Can you work these out from the model? Positions are in its coordinate system, mm. A direction names the side the tool comes from. Coordinates: 2 decimals unless noted, no trailing zeros. Write each loop counter-clockwise with the first axis right and the second up, starting at its lowest first coordinate (ties: lowest second). Pieces come first, ordered by that corner, then holes. Notation, with made-up numbers: (-22.75, -27) - (17.25, -27) arc R10 cw to (17.25, -12) - close; hole circle Ø1 at (40, -1.75). An arc over 180 degrees is marked (long way). Use one line per item in the form item = value. Start each with the question number.
(1) If we section it at D-D on y = -57.5: Please give me the cut outline in (x, z), then the cut area to 3 significant figures.
(2) If we section it at B-B on x = 67.5: Please give me the cut outline in (y, z).
(3) On a 3-axis mill with a long thin cutter (end or side, diameter ignored), from which of +Z, -Z, +X, -X, +Y, -Y can I reach the whole of each face in a straight line? I mean faces 5 (the face through (102.8, -44.07, 0.02)), 6 (the face through (88.89, -38.34, 0.02)), 7 (the face through (76.481, -76.275, 0.022)). Say none if no direction works.
(4) Thinking about a two-plate mould opening in Y: for faces 1 (the face through (22.77, -84.54, 0.02)), 2 (the face through (126.226, -25.71, 0.022)), 3 (the face through (121.068, -37.137, 0.022)), 4 (the face through (108, 19, 1.588)), which applies, pulls with the +Y half, pulls with the -Y half, needs draft (parallel to the pull), parting line crosses it, or undercut?
(5) If we section it at A-A on z = -0.25: Please give me the cut outline in (x, y), then the cut area to 3 significant figures.
(6) If I drill on probe 1 along Y at (x, z) = (52, 0); probe 2 along Y at (x, z) = (72.5, 0.25); probe 3 along X at (y, z) = (-55, 0.55), over which ranges is the centre line in solid material (lowest first)? Write a range as from..to.
(7) For pin 1 Ø1.5 at (x, z) = (19.5, 1) entering from +Y; pin 2 Ø1 at (y, z) = (135, 0) entering from -X; pin 3 Ø1 at (x, z) = (1, 0.5) entering from +Y; pin 4 Ø8 at (x, y) = (44.5, 114) entering from +Z, each with a flat end and sliding along its axis, tell me the tip position at first contact or that it passes through.
(8) If we section it at C-C on x = 84.5: Please give me the cut outline in (y, z).
```python
from build123d import *

# Parameters (mm, degrees)
BOSS_EXTRUDE1_DEPTH = 1.5875
SKETCH3_W           = 208.645691316
SKETCH3_H           = 383.026987577
CUT_EXTRUDE1_DEPTH  = 121.098895727
BOSS_EXTRUDE2_DEPTH = 1.5875
FILLET1_R           = 6.35
FILLET2_R           = 12.7
SKETCH6_W           = 3.302
SKETCH6_H           = 12.7
CUT_EXTRUDE2_DEPTH  = 4.175


with BuildPart() as part:
    # Sketch2 → Boss-Extrude1 (new body, symmetric)
    with BuildSketch(Plane.XY):
        with BuildLine():
            ThreePointArc((-120.098895727, 19.05), (0.406748907, 139.2017743), (120.203613722, 18.343301545))
            ThreePointArc((120.203613722, 18.343301545), (101.067699546, -47.629728931), (50.138751442, -93.726))
            ThreePointArc((50.138751442, -93.726), (0.040174098, -101.514794876), (-50.058403246, -93.726))
            ThreePointArc((-50.058403246, -93.726), (-101.163912713, -47.327889321), (-120.098895727, 19.05))
        make_face()
        with BuildLine():
            ThreePointArc((-104.858895727, 19.05), (0.361930242, 123.961840203), (104.963877332, 18.432938489))
            ThreePointArc((104.963877332, 18.432938489), (88.446745877, -39.065849025), (44.40486057, -79.553359885))
            ThreePointArc((44.40486057, -79.553359885), (0.040463589, -86.274794876), (-44.323959374, -79.553531384))
            ThreePointArc((-44.323959374, -79.553531384), (-88.517658334, -38.801393502), (-104.858895727, 19.05))
        make_face(mode=Mode.SUBTRACT)
    extrude(amount=BOSS_EXTRUDE1_DEPTH, both=True)

    # Sketch3 → Cut-Extrude1 (cut, through all)
    with BuildSketch(Plane(origin=(0, 0, 0), x_dir=(0, 0, -1), z_dir=(1, 0, 0))):
        with Locations((4.266053154, 20.866300598)):
            Rectangle(SKETCH3_W, SKETCH3_H)
    extrude(amount=-CUT_EXTRUDE1_DEPTH, mode=Mode.SUBTRACT)

    # Sketch5 → Boss-Extrude2 (add, symmetric)
    with BuildSketch(Plane.XY):
        Polygon((106.258152496, -51.988683319), (130.011728615, -28.168431361), (114.573822099, -18.142937646), (100.046993583, -49.235229101), align=None)
    extrude(amount=BOSS_EXTRUDE2_DEPTH, both=True)

    # Fillet1
    fillet1_edges = [part.edges().sort_by_distance(p)[0] for p in [
        (100.046993583, -49.235229101, 0),
    ]]
    fillet(fillet1_edges, radius=FILLET1_R)

    # Fillet2
    fillet2_edges = [part.edges().sort_by_distance(p)[0] for p in [
        (114.573822099, -18.142937646, 0),
    ]]
    fillet(fillet2_edges, radius=FILLET2_R)

    # Sketch6 → Cut-Extrude2 (cut, through all)
    with BuildSketch(Plane.XY.offset(1.5875)):
        with Locations((1.651, 136.662280289)):
            Rectangle(SKETCH6_W, SKETCH6_H)
        Polygon((108.166218002, 79.740204673), (106.494925174, 82.588008087), (95.541835122, 76.159958748), (97.21312795, 73.312155334), align=None)
        Polygon((95.424252626, -39.741107061), (97.095545407, -36.89330362), (118.130209204, -49.237934313), (116.458916422, -52.085737754), align=None)
        with Locations((1.651, -98.974789488)):
            Rectangle(SKETCH6_W, SKETCH6_H)
    extrude(amount=-CUT_EXTRUDE2_DEPTH, mode=Mode.SUBTRACT)


solid = part.part
```
Reported:
q1.outline = (74.16, -1.59) - (94.22, -1.59) - (94.22, 1.59) - (74.16, 1.59) - close
q1.area = 63.7 mm2
q2.outline = (-83.33, -1.59) - (-63.89, -1.59) - (-63.89, 1.59) - (-83.33, 1.59) - close; (99.41, -1.59) - (118.49, -1.59) - (118.49, 1.59) - (99.41, 1.59) - close
q3.face_5 = +Z, -Z
q3.face_6 = +Z, -Z, -X
q3.face_7 = +Z, -Z, +X, -Y
q4.face_1 = undercut
q4.face_2 = pulls with the +Y half
q4.face_3 = pulls with the -Y half
q4.face_4 = needs draft
q5.outline = (0, -92.62) - (3.3, -92.62) - (3.3, -101.48) arc R165.01 ccw to (50.14, -93.73) arc R125.85 ccw to (97.14, -53.53) arc R6.35 cw to (104.9, -51.39) - (106.26, -51.99) - (109.96, -48.27) - (95.42, -39.74) - (97.1, -36.89) - (112.37, -45.86) - (130.01, -28.17) - (122.33, -23.18) arc R12.7 cw to (116.89, -9.63) arc R125.85 ccw to (120.2, 18.34) arc R120.15 ccw to (104.86, 77.8) - (97.21, 73.31) - (95.54, 76.16) - (103.21, 80.66) arc R120.15 ccw to (3.3, 139.16) - (3.3, 130.31) - (0, 130.31) - (0, 123.96) arc R104.91 cw to (104.96, 18.43) arc R110.61 cw to (44.4, -79.55) arc R149.77 cw to (0, -86.27) - close
q5.area = 5,690 mm2
q6.probe_1 = -92.79..-75.32, 110.2..127.39
q6.probe_2 = -79.56..-59.2, 94.93..114.9
q6.probe_3 = 76.49..96.09
q7.pin_1 = 137.74
q7.pin_2 = 3.3
q7.pin_3 = 130.31
q7.pin_4 = 1.59
q8.outline = (-68.73, -1.59) - (-45.01, -1.59) - (-45.01, 1.59) - (-68.73, 1.59) - close; (81.3, -1.59) - (104.52, -1.59) - (104.52, 1.59) - (81.3, 1.59) - close
